Read the model definition and answer for the solid it produces. Units are mm, in the model's axes. A direction names the side the tool comes from. Coordinates: 2 decimals unless noted, no trailing zeros. Write each loop counter-clockwise with the first axis right and the second up, starting at its lowest first coordinate (ties: lowest second). Pieces come first, ordered by that corner, then holes. Notation, with made-up numbers: (12, 26.5) -> (68, 26.5) arc R11 ccw to (68, 35.5) -> close; hole circle Ø3 at (74.25, -7.75). An arc over 180 degrees is marked (long way). Write item = value, one per line. Start each with the question number.
1) Find the intervals of material crossed by line 1 along X through (y, z) = (16, 0); line 2 along Z through (x, y) = (0, 15.5); line 3 along Z through (x, y) = (3, 15.5), in increasing order. Write a range as from..to.
2) For a pull along Z with two mould halves and no side action, classify faces 1 (the face through (10.44, 25.52, 3.29)), 2 (the face through (-6, 9, 6)), 3 (the face through (6, 36.05, -6)) as released by +Z, released by -Z, zero draft, split by the parting line, or undercut.
3) A tool of negligible diameter and unlimited length cuts with its end or side. For faces 4 (the face through (-2.46, 0, 13.04)), 5 (the face through (-10.298, 4.437, -7.896)), from which of +Z, -Z, +X, -X, +Y, -Y can it reach the whole face along a straight path? Write none if from no direction.
4) Flat-ended cylindrical pins translate along their axes: pin 1 Ø3 at (y, z) = (20, 2) entering from -X; pin 2 Ø2 at (x, y) = (-10.5, 16.5) entering from +Z; pin 3 Ø4 at (x, y) = (-8, 20.5) entering from +Z; pin 4 Ø12.5 at (x, z) = (0, 0) entering from -Y. Find the tip coordinate at first contact, or state that the pin passes through.
5) Section B-B (y = 33) is taken. Determine the outline of the cut face in (x, z).
6) Section A-A (y = 27.5) is taken. Determine the outline of the cut face in (x, z).
Autodesk Inventor part; units mm, degrees
ref_plane "YZ Plane" through (0, 0, 0) normal (1, 0, 0) x (0, 1, 0)
ref_plane "XZ Plane" through (0, 0, 0) normal (0, 1, 0) x (-1, 0, 0)
ref_plane "XY Plane" through (0, 0, 0) normal (0, 0, 1) x (1, 0, 0)
sketch "Sketch2" plane through (0, 0, 0) normal (0, 0, 1) x (1, 0, 0)
  line L0 (12.85, 9) -> (13.1, 0)
  line L1 (0, 0) -> (13.1, 0) construction
  line L2 (0, 9) -> (12.85, 9) construction
  line L3 (0, 0) -> (0, 9) construction
  line L4 (16.1, 0) -> (16.1, 9)
  line L5 (16.1, 9) -> (11.05, 14.05)
  line L6 (11.05, 14.05) -> (10.85, 36.05)
  line L7 (10.85, 36.05) -> (7.85, 36.05)
  line L8 (7.85, 36.05) -> (7.85, 9)
  line L9 (7.85, 9) -> (12.85, 9)
  line L10 (13.1, 0) -> (16.1, 0)
  line L11 (0, -7.21) -> (0, 43.26)
  dimension "d0" = 13.1
  dimension "d1" = 12.85
  dimension "d2" = 9
  dimension "d3" = 3
  dimension "d4" = 45
  dimension "d5" = 11.05
  dimension "d6" = 22
  dimension "d7" = 10.85
  dimension "d8" = 3
revolve "Revolution1" add sketch "Sketch2" angle 360 about axis through (0, -10, 0) along (0, 1, 0)
fillet "Fillet2" radius 3 2 edges at (-11.05, 14.05, 0) (-16.1, 9, 0)
properties part number "BlowerInletPort_3DPrint"
Answer key:
q1.line_1 = -11.03..-7.85, 7.85..11.03
q1.line_2 = -11.04..-7.85, 7.85..11.04
q1.line_3 = -10.62..-7.25, 7.25..10.62
q2.face_1 = split by the parting line
q2.face_2 = undercut
q2.face_3 = zero draft
q3.face_4 = +Z, -Z, +X, -X, -Y
q3.face_5 = -Y
q4.pin_1 = -10.99
q4.pin_2 = 5.6
q4.pin_3 = 9.21
q4.pin_4 = through
q5.outline = circle Ø21.76 at (0, 0); hole circle Ø15.7 at (0, 0)
q6.outline = circle Ø21.86 at (0, 0); hole circle Ø15.7 at (0, 0)
